The listing builds one solid part. Answer for the finished solid, in the listing's coordinates (mm). Face numbers are marked on the shaded views. A direction names the side the tool comes from. Give positions to 0.01 mm unless a question says otherwise; leave off trailing zeros. Order: outer loops, then holes, each group sorted by start corner. A loop starts at its lowest first (then second) coordinate and runs counter-clockwise, first axis right, second up. Notation, with made-up numbers: (-19, 12) - (37, 12) arc R16 cw to (37, 23) - close; hole circle Ø6 at (19, -30.75). An arc over 180 degrees is marked (long way). Use a Markdown table: item, result. Add a question column.
1) Find section B-B, the plane x = -37.5. Determine the outline of the cut face in (y, z), plus the area to 3 significant figures.
2) Flat-ended cylindrical pins translate along their axes: pin 1 (8.5 mm diameter, centred on x = 37.5, y = 0, fed in from +Z); pin 2 (5.5 mm diameter, centred on x = -37.5, y = 0, fed in from -Z); pin 3 (3 mm diameter, centred on x = -29, y = 1, fed in from -Z); pin 4 (11 mm diameter, centred on x = -37.5, y = 0, fed in from -Z). Find the tip coordinate at first contact, or state that the pin passes through.
3) Find section A-A, the plane z = -16.75. Determine the outline of the cut face in (x, y).
4) For the marked faces 5 and 6, determine the directions among +Z, -Z, +X, -X, +Y, -Y from which every point of the face is accessible in a straight line to the end or side of a thin tool.
5) Find section D-D, the plane y = 0. Determine the outline of the cut face in (x, z).
6) Find section C-C, the plane y = -10.5. Determine the outline of the cut face in (x, z), plus the area to 3 significant figures.
7) Straight lines are drawn through the part: line 1 (X direction, y = 0, z = -7.5); line 2 (Y direction, x = -37.5, z = -5.25); line 3 (X direction, y = 0, z = -18.25). For each, find the intervals that lie inside material, in ascending order.
8) The mould has two halves that part along X. Classify the marked faces 1, 2, 3 and 4: released by +X, released by -X, zero draft, split by the parting line, or undercut.
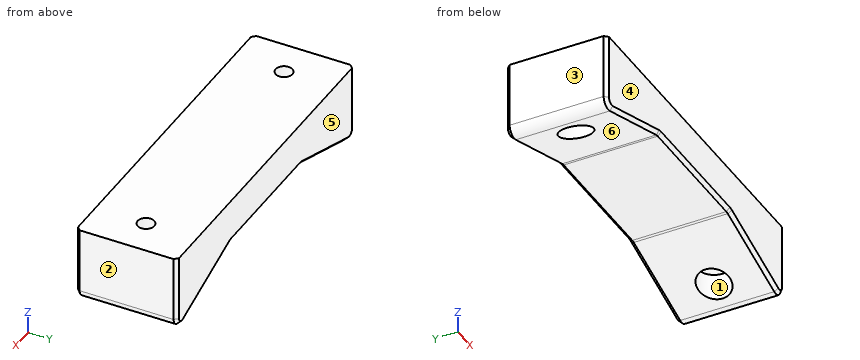
from build123d import *

# Parameters (mm, degrees)
BOSS_EXTRUDE1_DEPTH                            = 14.5
CSK_FOR_M4_FLAT_HEAD_MACHINE_SCREW1_AT_2_COUNT = 2
CSK_FOR_M4_FLAT_HEAD_MACHINE_SCREW1_AT_2_PITCH = 75
FILLET1_R                                      = 2.54
CHAMFER1_SIZE                                  = 1.016


with BuildPart() as part:
    # Sketch1 → Boss-Extrude1 (new, symmetric)
    with BuildSketch(Plane(origin=(0, 0, 0), x_dir=(1, 0, 0), z_dir=(0, 1, 0))):
        Polygon((-48, 0), (48, 0), (48, 22.35), (19.05, 12.7), (-19.05, 12.7), (-48, 22.35), align=None)
    extrude(amount=BOSS_EXTRUDE1_DEPTH, both=True)

    # Sketch5 → CSK for M4 Flat Head Machine Screw1 (revolve, cut)
    with BuildSketch(Plane(origin=(-37.5, 0, -25.4), x_dir=(0, 1, 0), z_dir=(1, 0, 0))):
        Polygon((0, 0), (0, 25.4), (2.4, 25.4), (2.4, 15), (4.7, 12.7), (4.7, 0), align=None)
    csk_for_m4_flat_head_machine_screw1 = revolve(axis=Axis((-37.5, 0, -31.75), (0, 0, 1)), mode=Mode.SUBTRACT)

    # CSK for M4 Flat Head Machine Screw1 at 2: CSK for M4 Flat Head Machine Screw1 ×2
    with Locations(*[(i * CSK_FOR_M4_FLAT_HEAD_MACHINE_SCREW1_AT_2_PITCH, 0, 0) for i in range(1, CSK_FOR_M4_FLAT_HEAD_MACHINE_SCREW1_AT_2_COUNT)]):
        add(csk_for_m4_flat_head_machine_screw1, mode=Mode.SUBTRACT)

    # Fillet1
    fillet1_edges = [part.edges().sort_by_distance(p)[0] for p in [
        (-48, 0, -22.35),
        (-19.05, 0, -12.7),
        (19.05, 0, -12.7),
        (48, 0, -22.35),
    ]]
    fillet(fillet1_edges, radius=FILLET1_R)

    # Chamfer1
    chamfer1_edges = [part.edges().sort_by_distance(p)[0] for p in [
        (-48, -14.5, -9.412969124),
        (-48, 14.5, -9.412969124),
        (-32.048907372, -14.5, -17.032969124),
        (0, -14.5, -12.7),
        (32.048907372, -14.5, -17.032969124),
        (46.945164123, -14.5, -20.886493398),
        (-46.945164123, -14.5, -20.886493398),
        (-32.048907372, 14.5, -17.032969124),
        (32.048907372, 14.5, -17.032969124),
        (0, 14.5, -12.7),
        (46.945164123, 14.5, -20.886493398),
        (-46.945164123, 14.5, -20.886493398),
        (-19.04467764, -14.5, -12.732797858),
        (-19.04467764, 14.5, -12.732797858),
        (19.04467764, -14.5, -12.732797858),
        (19.04467764, 14.5, -12.732797858),
        (48, 14.5, -9.412969124),
        (48, -14.5, -9.412969124),
    ]]
    chamfer(chamfer1_edges, length=CHAMFER1_SIZE)


solid = part.part
The answers:
| question | item | result |
|---|---|---|
| 1 | outline | (-14.5, -17.78) - (-13.48, -18.85) - (-4.7, -18.85) - (-4.7, -12.7) - (-2.4, -10.4) - (-2.4, 0) - (-14.5, 0) - close; (2.4, -10.4) - (4.7, -12.7) - (4.7, -18.85) - (13.48, -18.85) - (14.5, -17.78) - (14.5, 0) - (2.4, 0) - close |
| 1 | area | 422 mm2 |
| 2 | pin 1 | z = 0 |
| 2 | pin 2 | z = -10.75 |
| 2 | pin 3 | z = -16.52 |
| 2 | pin 4 | z = -20.68 |
| 3 | outline | (-48, -13.48) - (-46.98, -14.5) - (-34.41, -14.5) - (-31.2, -13.48) - (-31.2, 13.48) - (-34.41, 14.5) - (-46.98, 14.5) - (-48, 13.48) - close; (31.2, -13.48) - (34.41, -14.5) - (46.98, -14.5) - (48, -13.48) - (48, 13.48) - (46.98, 14.5) - (34.41, 14.5) - (31.2, 13.48) - close; hole circle Ø9.4 at (-37.5, 0); hole circle Ø9.4 at (37.5, 0) |
| 4 | face 5 | +Z, -Z, +X, -X, +Y |
| 4 | face 6 | -Z, +Y, -Y |
| 5 | outline | (-48, -18.83) arc R2.54 ccw to (-44.66, -21.24) - (-42.2, -20.42) - (-42.2, -12.7) - (-39.9, -10.4) - (-39.9, 0) - (-48, 0) - close; (-35.1, -10.4) - (-32.8, -12.7) - (-32.8, -17.28) - (-19.44, -12.83) arc R2.54 cw to (-18.64, -12.7) - (18.64, -12.7) arc R2.54 cw to (19.44, -12.83) - (32.8, -17.28) - (32.8, -12.7) - (35.1, -10.4) - (35.1, 0) - (-35.1, 0) - close; (39.9, -10.4) - (42.2, -12.7) - (42.2, -20.42) - (44.66, -21.24) arc R2.54 ccw to (48, -18.83) - (48, 0) - (39.9, 0) - close |
| 6 | outline | (-48, -18.83) arc R2.54 ccw to (-44.66, -21.24) - (-19.44, -12.83) arc R2.54 cw to (-18.64, -12.7) - (18.64, -12.7) arc R2.54 cw to (19.44, -12.83) - (44.66, -21.24) arc R2.54 ccw to (48, -18.83) - (48, 0) - (-48, 0) - close |
| 6 | area | 1,490 mm2 |
| 7 | line 1 | -48 to -39.9, -35.1 to 35.1, 39.9 to 48 |
| 7 | line 2 | -14.5 to -2.4, 2.4 to 14.5 |
| 7 | line 3 | -48 to -42.2, 42.2 to 48 |
| 8 | face 1 | undercut |
| 8 | face 2 | released by +X |
| 8 | face 3 | released by -X |
| 8 | face 4 | zero draft |
